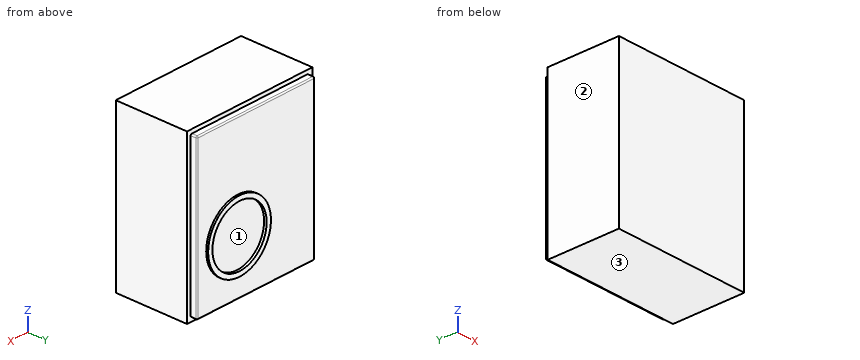
```python
from build123d import *

# Parameters (mm, degrees)
SKETCH1_W           = 270
SKETCH1_H           = 320
BOSS_EXTRUDE1_DEPTH = 142
SKETCH3_W           = 254
SKETCH3_H           = 304.8
BOSS_EXTRUDE3_DEPTH = 12.7
FILLET1_R           = 2.54
FILLET2_R           = 2.54
SKETCH7_R           = 67.678561976
BOSS_EXTRUDE4_DEPTH = 3.81
SKETCH8_R           = 58.425044715
CUT_EXTRUDE2_DEPTH  = 5.08


with BuildPart() as part:
    # Sketch1 → Boss-Extrude1 (new body)
    with BuildSketch(Plane(origin=(0, 0, 0), x_dir=(1, 0, 0), z_dir=(0, 1, 0))):
        Rectangle(SKETCH1_W, SKETCH1_H)
    extrude(amount=BOSS_EXTRUDE1_DEPTH)

    # Sketch3 → Boss-Extrude3 (add)
    with BuildSketch(Plane(origin=(0, 142, 0), x_dir=(1, 0, 0), z_dir=(0, 1, 0))):
        Rectangle(SKETCH3_W, SKETCH3_H)
    extrude(amount=BOSS_EXTRUDE3_DEPTH)

    # Fillet1
    fillet1_edges = [part.edges().sort_by_distance(p)[0] for p in [
        (127, 148.35, 152.4),
        (127, 148.35, -152.4),
        (-127, 148.35, -152.4),
        (-127, 148.35, 152.4),
    ]]
    fillet(fillet1_edges, radius=FILLET1_R)

    # Fillet2
    fillet2_edges = [part.edges().sort_by_distance(p)[0] for p in [
        (0, 154.7, -152.4),
        (127, 154.7, 0),
        (-127, 154.7, 0),
        (0, 154.7, 152.4),
        (126.256051224, 154.7, 151.656051224),
        (-126.256051224, 154.7, 151.656051224),
        (-126.256051224, 154.7, -151.656051224),
        (126.256051224, 154.7, -151.656051224),
    ]]
    fillet(fillet2_edges, radius=FILLET2_R)

    # Sketch7 → Boss-Extrude4 (add)
    with BuildSketch(Plane(origin=(0, 154.7, 0), x_dir=(1, 0, 0), z_dir=(0, 1, 0))):
        with Locations((39.597638404, 45.550655758)):
            Circle(SKETCH7_R)
    extrude(amount=BOSS_EXTRUDE4_DEPTH)

    # Sketch8 → Cut-Extrude2 (cut)
    with BuildSketch(Plane(origin=(0, 158.51, 0), x_dir=(1, 0, 0), z_dir=(0, 1, 0))):
        with Locations((39.597638404, 45.550655758)):
            Circle(SKETCH8_R)
    extrude(amount=-CUT_EXTRUDE2_DEPTH, mode=Mode.SUBTRACT)


solid = part.part
```
Design review of the part built by this model. Coordinates are the model's own, in mm. Face numbers are marked on the shaded views. Round coordinates to 2 decimals unless told otherwise and drop trailing zeros. Write each loop counter-clockwise with the first axis right and the second up, starting at its lowest first coordinate (ties: lowest second). Pieces come first, ordered by that corner, then holes. Notation, with made-up numbers: (23, 40) -> (76, 40) arc R16 ccw to (76, 52) -> close; hole circle Ø3 at (89, 75). An arc over 180 degrees is marked (long way). Answer in a Markdown table with one row per item.
Q1. To check wall thickness, follow L1, parallel to Y at x = -3, z = 59.5; L2, parallel to Z at x = 1, y = 145.5; L3, parallel to Y at x = 13, z = -64.5. State the ranges of each line that lie inside material, in increasing order. Write a range as [from, to].
The answers:
| item | result |
|---|---|
| L1 | [0, 154.7] |
| L2 | [-152.4, 152.4] |
| L3 | [0, 153.43] |
Q2. Clearance check with flat-ended pins moving along their axes: pin 1 Ø1.5 at (x, z) = (-71, -11.5) entering from -Y; pin 2 Ø8 at (x, y) = (-7, 149.5) entering from +Z; pin 3 Ø3 at (y, z) = (146.5, -58.5) entering from -X; pin 4 Ø3 at (x, z) = (13.5, 101.5) entering from +Y. State where each tip first meets the part, or that it passes through.
The answers:
| item | result |
|---|---|
| pin 1 | y = 0 |
| pin 2 | z = 152.4 |
| pin 3 | x = -127 |
| pin 4 | y = 154.7 |
Q3. Take a section at B-B, the plane x = -95. State the section outline as (y, z) points, then the cut area to 3 significant figures.
The answers:
| item | result |
|---|---|
| outline | (0, -160) -> (142, -160) -> (142, -152.4) -> (152.16, -152.4) arc R2.54 ccw to (154.7, -149.86) -> (154.7, 149.86) arc R2.54 ccw to (152.16, 152.4) -> (142, 152.4) -> (142, 160) -> (0, 160) -> close |
| area | 49,300 mm² |
Q4. Take a section at C-C, the plane z = 4.5. State the section outline as (x, y) points, then the cut area to 3 significant figures.
The answers:
| item | result |
|---|---|
| outline | (-135, 0) -> (135, 0) -> (135, 142) -> (127, 142) -> (127, 152.16) arc R2.54 ccw to (124.46, 154.7) -> (85.15, 154.7) -> (85.15, 158.51) -> (69.74, 158.51) -> (69.74, 153.43) -> (9.46, 153.43) -> (9.46, 158.51) -> (-5.96, 158.51) -> (-5.96, 154.7) -> (-124.46, 154.7) arc R2.54 ccw to (-127, 152.16) -> (-127, 142) -> (-135, 142) -> close |
| area | 41,600 mm² |
Q5. Take a section at A-A, the plane z = -140. State the section outline as (x, y) points, then the cut area to 3 significant figures.
The answers:
| item | result |
|---|---|
| outline | (-135, 0) -> (135, 0) -> (135, 142) -> (127, 142) -> (127, 152.16) arc R2.54 ccw to (124.46, 154.7) -> (-124.46, 154.7) arc R2.54 ccw to (-127, 152.16) -> (-127, 142) -> (-135, 142) -> close |
| area | 41,600 mm² |
Q6. Draft analysis for pull direction Z (two halves, no side actions). For the marked faces 1, 2 and 3, state which applies: +Z half, -Z half, draft (parallel to the pull), parting line (faces both ways), or undercut.
The answers:
| item | result |
|---|---|
| face 1 | undercut |
| face 2 | draft |
| face 3 | -Z half |
Q7. Take a section at D-D, the plane x = 70. State the section outline as (y, z) points.
The answers:
| item | result |
|---|---|
| outline | (0, -160) -> (142, -160) -> (142, -152.4) -> (152.16, -152.4) arc R2.54 ccw to (154.7, -149.86) -> (154.7, -106.02) -> (158.51, -106.02) -> (158.51, -95.44) -> (153.43, -95.44) -> (153.43, 4.34) -> (158.51, 4.34) -> (158.51, 14.91) -> (154.7, 14.91) -> (154.7, 149.86) arc R2.54 ccw to (152.16, 152.4) -> (142, 152.4) -> (142, 160) -> (0, 160) -> close |
